```python
from build123d import *

# Parameters (mm, degrees)
F1_DEPTH             = 96
F3_DEPTH             = 40.001
F6_D                 = 3.3
F6_DEPTH             = 30
F6_CBORE_D           = 6.5
F6_CBORE_DEPTH       = 3
F6_TIP               = 0.9914200214
F6_ON_F4_D           = 3.3
F6_ON_F4_DEPTH       = 30
F6_ON_F4_CBORE_D     = 6.5
F6_ON_F4_CBORE_DEPTH = 3
F6_ON_F4_TIP         = 0.9914200214
F8_DEPTH             = 40.001
F10_DEPTH            = 3
F12_DEPTH            = 3
F14_DEPTH            = 3
F15_R                = 1.6
F15_R_2              = 12.6
F16_DEPTH            = 25
F17_R                = 10


with BuildPart() as f1:
    # F0 (on Front) → F1 (new body)
    with BuildSketch(Plane.XZ):
        with BuildLine():
            Line((0, 30), (0, 0))
            Line((0, 0), (40, 0))
            Line((40, 0), (40, 30))
            Line((40, 30), (32.6, 30))
            ThreePointArc((32.6, 30), (20, 17.4), (7.4, 30))
            Line((7.4, 30), (0, 30))
        make_face()
    extrude(amount=F1_DEPTH)

    # F2 (on face) → F3 (cut, through all)
    with BuildSketch(Plane.YZ.offset(40)):
        with BuildLine():
            Line((-87.25, 0), (-87.25, 8.0709415886))
            ThreePointArc((-87.25, 8.0709415886), (-88, 16), (-88.75, 8.0709415886))
            Line((-88.75, 8.0709415886), (-88.75, 0))
            Line((-88.75, 0), (-87.25, 0))
        make_face()
        with BuildLine():
            Line((-7.25, 0), (-7.25, 8.0709415886))
            ThreePointArc((-7.25, 8.0709415886), (-8, 16), (-8.75, 8.0709415886))
            Line((-8.75, 8.0709415886), (-8.75, 0))
            Line((-8.75, 0), (-7.25, 0))
        make_face()
    extrude(amount=-F3_DEPTH, mode=Mode.SUBTRACT)

    # F6
    with Locations(Plane.XZ.offset(96)):
        with Locations((8, 5), (32, 5)):
            CounterBoreHole(F6_D / 2, F6_CBORE_D / 2, F6_CBORE_DEPTH, depth=F6_DEPTH)
            with Locations((0, 0, -(F6_DEPTH + F6_TIP / 2))):  # 118° drill point
                Cone(0, F6_D / 2, F6_TIP, mode=Mode.SUBTRACT)

    # F6 on F4
    with Locations(Plane(origin=(0, 0, 0), x_dir=(-1, 0, 0), z_dir=(0, 1, 0))):
        with Locations((-8, 5), (-32, 5)):
            CounterBoreHole(F6_ON_F4_D / 2, F6_ON_F4_CBORE_D / 2, F6_ON_F4_CBORE_DEPTH, depth=F6_ON_F4_DEPTH)
            with Locations((0, 0, -(F6_ON_F4_DEPTH + F6_ON_F4_TIP / 2))):  # 118° drill point
                Cone(0, F6_ON_F4_D / 2, F6_ON_F4_TIP, mode=Mode.SUBTRACT)

    # F7 (on face) → F8 (cut, through all)
    with BuildSketch(Plane(origin=(0, 0, 0), x_dir=(0, -1, 0), z_dir=(-1, 0, 0))):
        with BuildLine():
            Line((18, 11), (18, 0))
            Line((18, 0), (78, 0))
            Line((78, 0), (78, 11))
            ThreePointArc((78, 11), (76.5355339059, 14.5355339059), (73, 16))
            Line((73, 16), (23, 16))
            ThreePointArc((23, 16), (19.4644660941, 14.5355339059), (18, 11))
        make_face()
    extrude(amount=-F8_DEPTH, mode=Mode.SUBTRACT)

    # F9 (on face) → F10 (cut)
    with BuildSketch(Plane(origin=(0, 0, 16), x_dir=(1, 0, 0), z_dir=(0, 0, -1))):
        Polygon((7.5, 66.2679491924), (7.5, 69.7320508076), (4.5, 71.4641016151), (1.5, 69.7320508076), (1.5, 66.2679491924), (4.5, 64.5358983849), align=None)
        Polygon((32.5, 69.7320508076), (32.5, 66.2679491924), (35.5, 64.5358983849), (38.5, 66.2679491924), (38.5, 69.7320508076), (35.5, 71.4641016151), align=None)
        Polygon((7.5, 26.2679491924), (7.5, 29.7320508076), (4.5, 31.4641016151), (1.5, 29.7320508076), (1.5, 26.2679491924), (4.5, 24.5358983849), align=None)
        Polygon((32.5, 29.7320508076), (32.5, 26.2679491924), (35.5, 24.5358983849), (38.5, 26.2679491924), (38.5, 29.7320508076), (35.5, 31.4641016151), align=None)
    extrude(amount=-F10_DEPTH, mode=Mode.SUBTRACT)

    # F11 (on face) → F12 (cut)
    with BuildSketch(Plane.XZ.offset(18)):
        Polygon((11, 3.2679491924), (11, 6.7320508076), (8, 8.4641016151), (5, 6.7320508076), (5, 3.2679491924), (8, 1.5358983849), align=None)
        Polygon((35, 3.2679491924), (35, 6.7320508076), (32, 8.4641016151), (29, 6.7320508076), (29, 3.2679491924), (32, 1.5358983849), align=None)
    extrude(amount=-F12_DEPTH, mode=Mode.SUBTRACT)

    # F13 (on face) → F14 (cut)
    with BuildSketch(Plane(origin=(0, -78, 0), x_dir=(-1, 0, 0), z_dir=(0, 1, 0))):
        Polygon((-35, 6.7320508076), (-35, 3.2679491924), (-32, 1.5358983849), (-29, 3.2679491924), (-29, 6.7320508076), (-32, 8.4641016151), align=None)
        Polygon((-11, 6.7320508076), (-11, 3.2679491924), (-8, 1.5358983849), (-5, 3.2679491924), (-5, 6.7320508076), (-8, 8.4641016151), align=None)
    extrude(amount=-F14_DEPTH, mode=Mode.SUBTRACT)

    # F15 (on face) → F16 (cut)
    with BuildSketch(Plane.XY.offset(30)):
        with Locations((4.5, -28)):
            Circle(F15_R)
        with Locations((35.5, -28)):
            Circle(F15_R)
        with Locations((35.5, -68)):
            Circle(F15_R)
        with Locations((4.5, -68)):
            Circle(F15_R)
        with Locations((20, -48)):
            Circle(F15_R_2)
    extrude(amount=-F16_DEPTH, mode=Mode.SUBTRACT)

    # F17
    f17_edges = [f1.edges().sort_by_distance(p)[0] for p in [
        (36.3, -96, 30),
        (3.7, -96, 30),
        (3.7, 0, 30),
        (36.3, 0, 30),
    ]]
    fillet(f17_edges, radius=F17_R)


solid = f1.part
```
Can you work these out from the model? Positions are in its coordinate system, mm. A direction names the side the tool comes from. Round coordinates to 2 decimals unless told otherwise and drop trailing zeros. Loops run counter-clockwise (first coordinate to the right, second up) from the corner with the lowest first, then second, coordinate; pieces in that order, holes last. Notation, with made-up numbers: (-24, 64.5) -> (29, 64.5) arc R17 cw to (29, 72.5) -> close; hole circle Ø11 at (67.5, -18.5). An arc over 180 degrees is marked (long way). Answer in a Markdown table with one row per item.
Item 1: We'd pull the mould along Z, two halves only. Please class faces 1 (the flat face through (34, -25.4, 17.5)), 2 (the flat face through (3, -29, 19)), 3 (the flat face through (6.6, -3, 3.6)), 4 (the cylindrical face through (7.6, -5.2, 3.4)): released by +Z, released by -Z, zero draft, split by the parting line, or undercut.
Answer block:
| item | result |
|---|---|
| face 1 | zero draft |
| face 2 | released by -Z |
| face 3 | undercut |
| face 4 | undercut |
Item 2: Suppose I cut it at C-C, the plane y = -59. List the corners of the cut face in (x, z) for me, plus the area to 3 significant figures.
Answer block:
| item | result |
|---|---|
| outline | (0, 16) -> (13.86, 16) -> (13.86, 19) arc R12.6 cw to (7.4, 30) -> (0, 30) -> close; (26.14, 16) -> (40, 16) -> (40, 30) -> (32.6, 30) arc R12.6 cw to (26.14, 19) -> close |
| area | 287 mm² |
Item 3: Suppose I cut it at A-A, the plane y = -28. List the corners of the cut face in (x, z) for me, plus the area to 3 significant figures.
Answer block:
| item | result |
|---|---|
| outline | (0, 16) -> (1.5, 16) -> (1.5, 19) -> (2.9, 19) -> (2.9, 30) -> (0, 30) -> close; (6.1, 19) -> (7.5, 19) -> (7.5, 16) -> (32.5, 16) -> (32.5, 19) -> (33.9, 19) -> (33.9, 30) -> (32.6, 30) arc R12.6 cw to (7.4, 30) -> (6.1, 30) -> close; (37.1, 19) -> (38.5, 19) -> (38.5, 16) -> (40, 16) -> (40, 30) -> (37.1, 30) -> close |
| area | 204 mm² |
Item 4: On a 3-axis mill with a long thin cutter (end or side, diameter ignored), from which of +Z, -Z, +X, -X, +Y, -Y can I reach the whole of each face in a straight line? I mean faces 5 (the flat face through (20, -18, 6)), 6 (the cylindrical face through (4.292, -26.414, 24.577)), 7 (the flat face through (6, -70.6, 17.5)), 8 (the flat face through (35, -79, 5)). Say none if no direction works.
Answer block:
| item | result |
|---|---|
| face 5 | -Z, +X, -X |
| face 6 | +Z, -Z |
| face 7 | -Z |
| face 8 | none |
Item 5: Suppose I cut it at B-B, the plane z = 12. List the corners of the cut face in (x, y) for me.
Answer block:
| item | result |
|---|---|
| outline | (0, -96) -> (40, -96) -> (40, -92) -> (0, -92) -> close; (0, -84) -> (40, -84) -> (40, -77.9) -> (0, -77.9) -> close; (0, -18.1) -> (40, -18.1) -> (40, -12) -> (0, -12) -> close; (0, -4) -> (40, -4) -> (40, 0) -> (0, 0) -> close |
Item 6: Suppose I cut it at D-D, the plane x = 25.5. List the corners of the cut face in (y, z) for me, plus the area to 3 significant figures.
Answer block:
| item | result |
|---|---|
| outline | (-96, 0) -> (-88.75, 0) -> (-88.75, 8.07) arc R4 cw (long way) to (-87.25, 8.07) -> (-87.25, 0) -> (-78, 0) -> (-78, 11) arc R5 cw to (-73, 16) -> (-59.34, 16) -> (-59.34, 18.66) -> (-96, 18.66) -> close; (-36.66, 16) -> (-23, 16) arc R5 cw to (-18, 11) -> (-18, 0) -> (-8.75, 0) -> (-8.75, 8.07) arc R4 cw (long way) to (-7.25, 8.07) -> (-7.25, 0) -> (0, 0) -> (0, 18.66) -> (-36.66, 18.66) -> close |
| area | 657 mm² |
Item 7: Will these pins go through, and if not, where does the flat tip stop? P1, Ø3, axis at x = 31.5, z = 5.5, coming from the -Y side; P2, Ø6.5, axis at x = 5, y = -29, coming from the -Z side; P3, Ø5, axis at x = 4.5, y = -67.5, coming from the -Z side.
Answer block:
| item | result |
|---|---|
| P1 | y = -93 |
| P2 | z = 16 |
| P3 | z = 19 |
Item 8: If I drill on probe 1 along Y at (x, z) = (12, 4); probe 2 along Y at (x, z) = (35, 22.5); probe 3 along Y at (x, z) = (5, 28.5), over which ranges is the centre line in solid material (lowest first)?
Answer block:
| item | result |
|---|---|
| probe 1 | -96 to -88.75, -87.25 to -78, -18 to -8.75, -7.25 to 0 |
| probe 2 | -95.68 to -69.52, -66.48 to -29.52, -26.48 to -0.32 |
| probe 3 | -91.27 to -69.52, -66.48 to -29.52, -26.48 to -4.73 |
